```python
from build123d import *

# Parameters (mm, degrees)
CROQUIS1_W              = 89.34
CROQUIS1_H              = 89.34
SALIENTE_EXTRUIR2_DEPTH = 10
CROQUIS3_R              = 34.67
CORTAR_EXTRUIR2_DEPTH   = 10
CROQUIS4_R              = 5
CORTAR_EXTRUIR3_DEPTH   = 10
REDONDEO2_R             = 2


with BuildPart() as part:
    # Croquis1 → Saliente-Extruir2 (new body)
    with BuildSketch(Plane.XY):
        Rectangle(CROQUIS1_W, CROQUIS1_H)
    extrude(amount=SALIENTE_EXTRUIR2_DEPTH)

    # Croquis3 → Cortar-Extruir2 (cut)
    with BuildSketch(Plane.XY.offset(10)):
        Circle(CROQUIS3_R)
    extrude(amount=-CORTAR_EXTRUIR2_DEPTH, mode=Mode.SUBTRACT)

    # Croquis4 → Cortar-Extruir3 (cut)
    with BuildSketch(Plane.XY.offset(10)):
        with Locations((37.67, -37.67)):
            Circle(CROQUIS4_R)
        with Locations(Location((-37.67, -37.67, 0), (0, 0, 180))):
            Circle(CROQUIS4_R)
        with Locations((-37.67, 37.67)):
            Circle(CROQUIS4_R)
        with Locations(Location((37.67, 37.67, 0), (0, 0, 180))):
            Circle(CROQUIS4_R)
    extrude(amount=-CORTAR_EXTRUIR3_DEPTH, mode=Mode.SUBTRACT)

    # Redondeo2
    redondeo2_edges = [part.edges().sort_by_distance(p)[0] for p in [
        (-44.67, -44.67, 5),
        (-44.67, 44.67, 5),
        (44.67, 44.67, 5),
        (44.67, -44.67, 5),
    ]]
    fillet(redondeo2_edges, radius=REDONDEO2_R)


solid = part.part
```
Geometry: final body of the model. Coordinates: model frame, mm. Coordinates: 2 decimals unless noted, no trailing zeros. Order: outer loops, then holes, each group sorted by start corner. A loop starts at its lowest first (then second) coordinate and runs counter-clockwise, first axis right, second up. Notation, with made-up numbers: M 0.5,28 L 17.5,28 A9 cw 17.5,32 Z; hole C -18.5,-39 d1. An arc over 180 degrees is marked long. Answer in a Markdown table with one row per item. Add a question column.
Q1. Mould query, pull axis Y, two halves, no side actions, for faces 1 (the cylindrical face through (-44.1, -44.07, 5.07)), 2 (the cylindrical face through (-33.051, 35.755, 5.07)), 3 (the cylindrical face through (44.07, 44.1, 5.07)), 4 (the cylindrical face through (-27.51, -21.1, 5.07)). Classes: released by +Y, released by -Y, zero draft, split by the parting line, or undercut.
Q2. Line query: L1, parallel to Y at x = -37.67, z = 4.25; L2, parallel to Y at x = 35, z = 1; L3, parallel to Y at x = 0, z = 3.25. Output: solid intervals per line, ascending.
Q3. Section query D-D on x = 0. Return the cut outline in (y, z).
Q4. Section query A-A on x = -37.67. Return the cut outline in (y, z).
Q5. Section query B-B on z = 4. Return the cut outline in (x, y).
Completed:
| question | item | result |
|---|---|---|
| 1 | face 1 | released by -Y |
| 1 | face 2 | undercut |
| 1 | face 3 | released by +Y |
| 1 | face 4 | undercut |
| 2 | L1 | y = -44.67 to -42.67, -32.67 to 32.67, 42.67 to 44.67 |
| 2 | L2 | y = -44.67 to -41.9, -33.44 to 33.44, 41.9 to 44.67 |
| 2 | L3 | y = -44.67 to -34.67, 34.67 to 44.67 |
| 3 | outline | M -44.67,0 L -34.67,0 L -34.67,10 L -44.67,10 Z; M 34.67,0 L 44.67,0 L 44.67,10 L 34.67,10 Z |
| 4 | outline | M -44.67,0 L -42.67,0 L -42.67,10 L -44.67,10 Z; M -32.67,0 L 32.67,0 L 32.67,10 L -32.67,10 Z; M 42.67,0 L 44.67,0 L 44.67,10 L 42.67,10 Z |
| 5 | outline | M -44.67,-42.67 A2 ccw -42.67,-44.67 L 42.67,-44.67 A2 ccw 44.67,-42.67 L 44.67,42.67 A2 ccw 42.67,44.67 L -42.67,44.67 A2 ccw -44.67,42.67 Z; hole C -37.67,-37.67 d10; hole C -37.67,37.67 d10; hole C 0,0 d69.34; hole C 37.67,-37.67 d10; hole C 37.67,37.67 d10 |
